Autodesk Inventor part; units mm, degrees
ref_plane "YZ Plane" through (0, 0, 0) normal (1, 0, 0) x (0, 1, 0)
ref_plane "XZ Plane" through (0, 0, 0) normal (0, 1, 0) x (-1, 0, 0)
ref_plane "XY Plane" through (0, 0, 0) normal (0, 0, 1) x (1, 0, 0)
sketch "Sketch1" plane through (0, 0, 0) normal (0, 0, 1) x (1, 0, 0)
  line L0 (21.15, -21.15) -> (-21.15, -21.15)
  line L1 (-21.15, -21.15) -> (-21.15, 21.15)
  line L2 (-21.15, 21.15) -> (21.15, 21.15)
  line L3 (21.15, 21.15) -> (21.15, -21.15)
  line L4 (21.15, -21.15) -> (-21.15, 21.15) construction
  line L5 (-21.15, -21.15) -> (21.15, 21.15) construction
  point P0 (0, 0)
  dimension "d0" = 42.3
extrude "Extrusion1" add sketch "Sketch1" along normal blind 38
sketch "Sketch2" plane through (0, 0, 0) normal (0, 0, -1) x (-1, 0, 0)
  line L0 (15.5, -15.5) -> (-15.5, -15.5)
  line L1 (-15.5, -15.5) -> (-15.5, 15.5)
  line L2 (-15.5, 15.5) -> (15.5, 15.5)
  line L3 (15.5, 15.5) -> (15.5, -15.5)
  line L4 (15.5, -15.5) -> (-15.5, 15.5) construction
  line L5 (-15.5, -15.5) -> (15.5, 15.5) construction
  point P0 (0, 0)
  dimension "d3" = 31
hole "Hole1" at (15.5, 15.5, 0) at (-15.5, 15.5, 0) at (-15.5, -15.5, 0) at (15.5, -15.5, 0) direction (0, 0, 1) diameter 2.459 end through all
sketch "Sketch3" plane through (0, 0, 0) normal (0, 0, -1) x (-1, 0, 0)
  circle A0 centre (0, 0) radius 11
  dimension "d11" = 22
extrude "Extrusion2" add sketch "Sketch3" along normal blind 2
sketch "Sketch4" plane through (0, 0, -2) normal (0, 0, -1) x (-1, 0, 0)
  circle A0 centre (0, 0) radius 2.5
  line L0 (-1.5, 2) -> (1.5, 2)
  dimension "d14" = 5
  dimension "d15" = 4.5
extrude "Extrusion3" add sketch "Sketch4" along normal blind 21.5 contours A0 L0 picked at (0.1119, 0.5076)
properties part number "NEMA17"
Build history of the part. All positions in model axes, mm. A direction names the side the tool comes from. Round coordinates to 2 decimals unless told otherwise and drop trailing zeros. Loops run counter-clockwise (first coordinate to the right, second up) from the corner with the lowest first, then second, coordinate; pieces in that order, holes last.
Item 1: Saw through at C-C (y = 0). List the corners of the cut face in (x, z), then the cut area to 3 significant figures.
Item 2: Which spindle directions (+Z, -Z, +X, -X, +Y, -Y) get a long thin tool onto all of the face, cutting with end or side? Do faces 4 (the face through (0, 2, -13)), 5 (the face through (2.38, 10.74, -0.99)), 6 (the face through (0, 0, -23.5)). Say none if no direction does.
Item 3: Pin check, flat tip, straight feed: P1, Ø1.5, axis at x = 0.5, z = -11, coming from the +Y side. Stop position of the tip, or through.
Item 4: Saw through at D-D (x = 10). List the corners of the cut face in (y, z), then the cut area to 3 significant figures.
Item 5: Two-plate mould, pull along X, no slides. Class faces 1 (the face through (0, 3, -2)), 2 (the face through (21.15, 0, 19)), 3 (the face through (15.131, 16.673, 19.266)): released by +X, released by -X, zero draft, split by the parting line, or undercut.
Item 6: Drill centre lines: line 1 along X through (y, z) = (15.5, 22); line 2 along X through (y, z) = (-15, 21). Where is each one in solid material? Low to high.
Item 7: Saw through at A-A (x = -15.5). List the corners of the cut face in (y, z).
Worked answers:
1. outline: (-21.15, 0) - (-11, 0) - (-11, -2) - (-2.5, -2) - (-2.5, -23.5) - (2.5, -23.5) - (2.5, -2) - (11, -2) - (11, 0) - (21.15, 0) - (21.15, 38) - (-21.15, 38) - close
1. area: 1,760 mm2
2. face 4: -Z, +X, -X, +Y
2. face 5: -Z
2. face 6: -Z, +X, -X, +Y, -Y
3. P1: stops at y = 2
4. outline: (-21.15, 0) - (-4.58, 0) - (-4.58, -2) - (4.58, -2) - (4.58, 0) - (21.15, 0) - (21.15, 38) - (-21.15, 38) - close
4. area: 1,630 mm2
5. face 1: zero draft
5. face 2: released by +X
5. face 3: undercut
6. line 1: x = -21.15 to -16.73, -14.27 to 14.27, 16.73 to 21.15
6. line 2: x = -21.15 to -16.62, -14.38 to 14.38, 16.62 to 21.15
7. outline: (-21.15, 0) - (-16.73, 0) - (-16.73, 38) - (-21.15, 38) - close; (-14.27, 0) - (14.27, 0) - (14.27, 38) - (-14.27, 38) - close; (16.73, 0) - (21.15, 0) - (21.15, 38) - (16.73, 38) - close
